Source: three-view drawing plus pictorial views. Frame: mm from the lowest corner of the part. A direction names the side the tool comes from. Give positions to 0.01 mm unless a question says otherwise; leave off trailing zeros. Loops run counter-clockwise (first coordinate to the right, second up) from the corner with the lowest first, then second, coordinate; pieces in that order, holes last. Notation, with made-up numbers: (-6.75, -7) - (26.25, -7) arc R25 ccw to (26.25, 30) - close; hole circle Ø3 at (-32.5, 76.5). An arc over 180 degrees is marked (long way). Put each result on its own line as item: value.
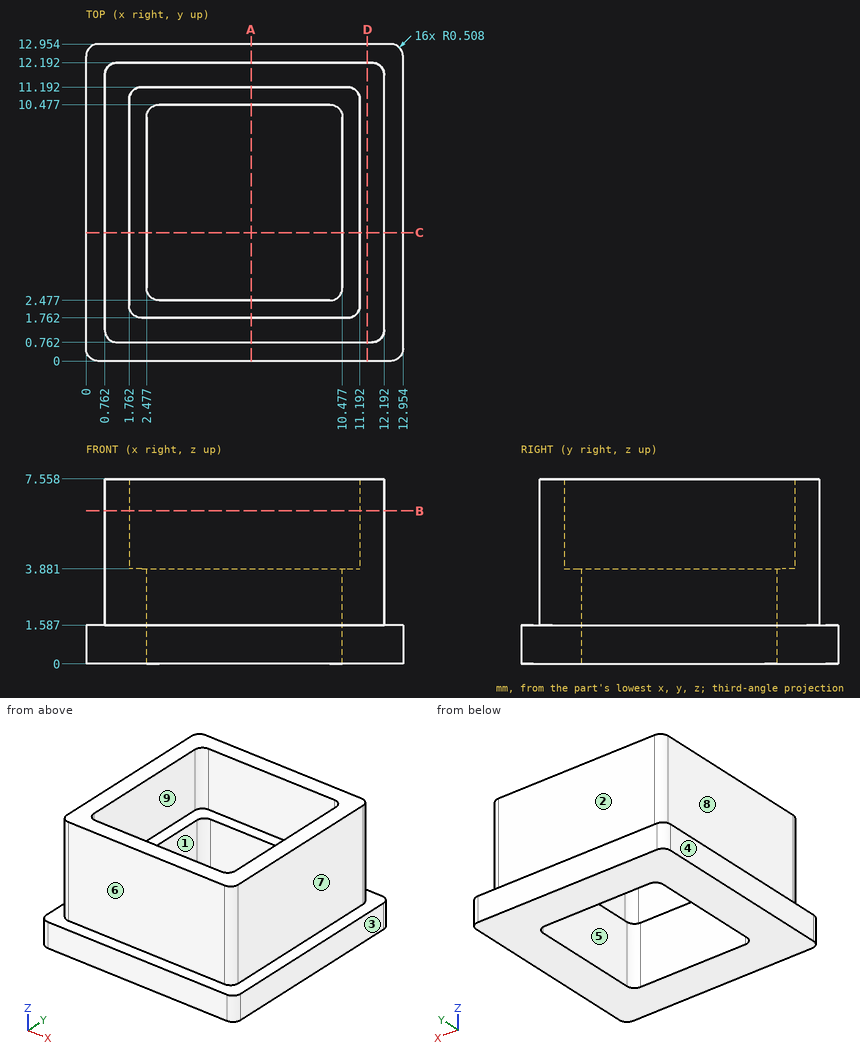
1) Material intervals for line 1 along Y through (x, z) = (3.5, 6.5); line 2 along Y through (x, z) = (9.75, 3.5), sorted ascending. Write a range as [from, to].
Check result:
line 1: [0.76, 1.76], [11.19, 12.19]
line 2: [0.76, 2.48], [10.48, 12.19]
2) Access query for the marked faces 5, 6, 7, 8 and 9. Directions: +Z, -Z, +X, -X, +Y, -Y. A direction counts if a zero-diameter tool reaches every point of the face in a straight line with its end or side. Return the directions, or none.
Check result:
face 5: +Z, -Z
face 6: +Z, +X, -X, -Y
face 7: +Z, +X, +Y, -Y
face 8: +Z, -X, +Y, -Y
face 9: +Z
3) Section query B-B, the plane z = 6.25. Output: boundary loops of the cut face in (x, y) (1 decimal).
Check result:
outline: (0.8, 1.3) arc R0.5 ccw to (1.3, 0.8) - (11.7, 0.8) arc R0.5 ccw to (12.2, 1.3) - (12.2, 11.7) arc R0.5 ccw to (11.7, 12.2) - (1.3, 12.2) arc R0.5 ccw to (0.8, 11.7) - close; hole (1.8, 2.3) arc R0.5 ccw to (2.3, 1.8) - (10.7, 1.8) arc R0.5 ccw to (11.2, 2.3) - (11.2, 10.7) arc R0.5 ccw to (10.7, 11.2) - (2.3, 11.2) arc R0.5 ccw to (1.8, 10.7) - close
4) Section query A-A, the plane x = 6.75. Output: boundary loops of the cut face in (y, z) (1 decimal).
Check result:
outline: (0, 0) - (2.5, 0) - (2.5, 3.9) - (1.8, 3.9) - (1.8, 7.6) - (0.8, 7.6) - (0.8, 1.6) - (0, 1.6) - close; (10.5, 0) - (13, 0) - (13, 1.6) - (12.2, 1.6) - (12.2, 7.6) - (11.2, 7.6) - (11.2, 3.9) - (10.5, 3.9) - close
5) Pin query (flat end, axial travel): P1, Ø3, axis at x = 6.5, z = 3, coming from the +Y side; P2, Ø2, axis at y = 5.5, z = 4, coming from the +X side; P3, Ø1.8, axis at y = 6, z = 5.5, coming from the -X side; P4, Ø4, axis at x = 8, z = 6, coming from the -Y side. Return the tip coordinate at first contact, or that it passes through.
Check result:
P1: y = 12.95
P2: x = 12.19
P3: x = 0.76
P4: y = 0.76
6) Section query D-D, the plane x = 11.5. Output: boundary loops of the cut face in (y, z) (1 decimal), plus the area to 3 significant figures.
Check result:
outline: (0, 0) - (13, 0) - (13, 1.6) - (12.2, 1.6) - (12.2, 7.6) - (0.8, 7.6) - (0.8, 1.6) - (0, 1.6) - close
area: 88.8 mm²
7) Mould query, pull axis X, two halves, no side actions, for the marked faces 1, 2, 3 and 4. Classes: pulls with the +X half, pulls with the -X half, needs draft (parallel to the pull), parting line crosses it, or undercut.
Check result:
face 1: undercut
face 2: needs draft
face 3: pulls with the +X half
face 4: pulls with the -X half
